Work out the finished part from the listing and answer in its coordinate system (mm). Face numbers are marked on the shaded views. A direction names the side the tool comes from. Give positions to 0.01 mm unless a question says otherwise; leave off trailing zeros. Write each loop counter-clockwise with the first axis right and the second up, starting at its lowest first coordinate (ties: lowest second). Pieces come first, ordered by that corner, then holes.
1) Find section A-A (x = -33.5). Determine the outline of the cut face in (y, z), plus the area to 3 significant figures.
2) Straight lines are drawn through the part: probe 1 along Z at (x, y) = (-30, 78.5); probe 2 along Y at (x, z) = (38, 15.5). For each, find the intervals that lie inside material, in ascending order.
3) Find section C-C (y = 17.5). Determine the outline of the cut face in (x, z).
4) Find section B-B (z = 47.5). Determine the outline of the cut face in (x, y), plus the area to 3 significant figures.
5) Given pin 1 Ø5 at (x, z) = (37.74, 65.04) entering from -Y; pin 2 Ø3 at (x, z) = (31.5, 28.5) entering from +Y, each flat-ended and moving along its own axis, determine where each tip first touches the part or whether it passes through.
6) A tool of negligible diameter and unlimited length cuts with its end or side. For the marked faces 1 and 2, from which of +Z, -Z, +X, -X, +Y, -Y can it reach the whole face along a straight path? Write none if from no direction.
```python
from build123d import *

# Parameters (mm, degrees)
F0_W     = 101.6
F0_H     = 152.4
F1_DEPTH = 6.35
F2_W     = 139.7
F2_H     = 76.2
F3_DEPTH = 50.8
F4_DEPTH = 63.5
F5_SIZE  = 5.08
F6_R     = 5.08
F7_R     = 3.175
F8_DEPTH = 12.7


with BuildPart() as f1:
    # F0 (on Front) → F1 (new body, symmetric)
    with BuildSketch(Plane.XZ):
        Rectangle(F0_W, F0_H)
    extrude(amount=F1_DEPTH, both=True)

    # F2 (on Right) → F3 (join, symmetric)
    with BuildSketch(Plane.YZ):
        with Locations((69.85, -38.1)):
            Rectangle(F2_W, F2_H)
    extrude(amount=F3_DEPTH, both=True)

    # F4 (cut): a face of the model
    f4_faces = [f1.faces().sort_by_distance(p)[0] for p in [
        (0, 73.025, 0),
    ]]
    extrude(f4_faces, amount=-F4_DEPTH, mode=Mode.SUBTRACT)

    # F5
    f5_edges = [f1.edges().sort_by_distance(p)[0] for p in [
        (0, 6.35, -63.5),
    ]]
    chamfer(f5_edges, length=F5_SIZE)

    # F6
    f6_edges = [f1.edges().sort_by_distance(p)[0] for p in [
        (0, -6.35, -76.2),
    ]]
    fillet(f6_edges, radius=F6_R)

    # F7 (on face) → F8 (cut)
    with BuildSketch(Plane(origin=(0, 6.35, 0), x_dir=(-1, 0, 0), z_dir=(0, 1, 0))):
        with Locations((-37.7415953271, 65.0431930406)):
            Circle(F7_R)
        with Locations((33.4293011874, 66.8958395785)):
            Circle(F7_R)
        with Locations((33.7640900696, -45.4423770942)):
            Circle(F7_R)
        with Locations((-37.7306027449, -47.1545040206)):
            Circle(F7_R)
    extrude(amount=-F8_DEPTH, mode=Mode.SUBTRACT)


solid = f1.part
```
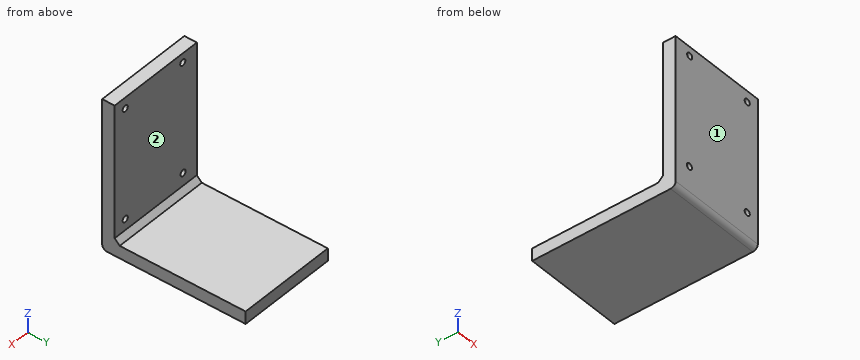
Results:
1. outline: (-6.35, -71.12) arc R5.08 ccw to (-1.27, -76.2) - (139.7, -76.2) - (139.7, -63.5) - (11.43, -63.5) - (6.35, -58.42) - (6.35, -48.61) - (-6.35, -48.61) - close; (-6.35, -42.28) - (6.35, -42.28) - (6.35, 63.72) - (-6.35, 63.72) - close; (-6.35, 70.07) - (6.35, 70.07) - (6.35, 76.2) - (-6.35, 76.2) - close
1. area: 3,480 mm2
2. probe 1: z = -76.2 to -63.5
2. probe 2: y = -6.35 to 6.35
3. outline: (-50.8, -76.2) - (50.8, -76.2) - (50.8, -63.5) - (-50.8, -63.5) - close
4. outline: (-50.8, -6.35) - (50.8, -6.35) - (50.8, 6.35) - (-50.8, 6.35) - close
4. area: 1,290 mm2
5. pin 1: passes through
5. pin 2: stops at y = 6.35
6. face 1: +Z, -Z, +X, -X, -Y
6. face 2: +Z, +X, -X, +Y
